from build123d import *

# Parameters (mm, degrees)
BOSS_EXTRU_1_DEPTH = 10
ESQUISSE2_R        = 10
BOSS_EXTRU_2_DEPTH = 110
CONG_1_R           = 2


with BuildPart() as part:
    # Esquisse1 → Boss.-Extru.1 (new body)
    with BuildSketch(Plane(origin=(0, 0, 0), x_dir=(1, 0, 0), z_dir=(0, 1, 0))):
        Polygon((14.736253584, 9.101803684), (-0.514266419, 17.312871803), (-15.250520003, 8.211068118), (-14.736253584, -9.101803684), (0.514266419, -17.312871803), (15.250520003, -8.211068118), align=None)
    extrude(amount=BOSS_EXTRU_1_DEPTH)

    # Esquisse2 → Boss.-Extru.2 (add)
    with BuildSketch(Plane(origin=(0, 10, 0), x_dir=(1, 0, 0), z_dir=(0, 1, 0))):
        Circle(ESQUISSE2_R)
    extrude(amount=BOSS_EXTRU_2_DEPTH)

    # Congé1
    cong_1_edges = [part.edges().sort_by_distance(p)[0] for p in [
        (-10, 120, 0),
    ]]
    fillet(cong_1_edges, radius=CONG_1_R)


solid = part.part
Can you work these out from the model? Positions are in its coordinate system, mm. A direction names the side the tool comes from. Coordinates: 2 decimals unless noted, no trailing zeros. Write each loop counter-clockwise with the first axis right and the second up, starting at its lowest first coordinate (ties: lowest second). Pieces come first, ordered by that corner, then holes. Notation, with made-up numbers: (-15, 31) -> (36, 31) arc R14 cw to (36, 43) -> close; hole circle Ø8 at (25.5, 66.5). An arc over 180 degrees is marked (long way). Write item = value, one per line.
(1) For pin 1 (1.5 mm diameter, centred on y = 80, z = -2, fed in from +X); pin 2 (2 mm diameter, centred on y = 63, z = -8, fed in from +X); pin 3 (12 mm diameter, centred on x = -5, y = 34, fed in from -Z), each with a flat end and sliding along its axis, tell me the tip position at first contact or that it passes through.
Verdict:
pin_1 = 9.92
pin_2 = 7.14
pin_3 = -10
(2) Imagine slicing it at B-B (z = 0). Please give me the cut outline in (x, y), and give its area (3 significant figures).
Verdict:
outline = (-15.01, 0) -> (15.01, 0) -> (15.01, 10) -> (10, 10) -> (10, 118) arc R2 ccw to (8, 120) -> (-8, 120) arc R2 ccw to (-10, 118) -> (-10, 10) -> (-15.01, 10) -> close
area = 2,500 mm^2
(3) Imagine slicing it at C-C (x = -13). Please give me the cut outline in (y, z), and give its area (3 significant figures).
Verdict:
outline = (0, -9.6) -> (10, -9.6) -> (10, 10.04) -> (0, 10.04) -> close
area = 196 mm^2
(4) Imagine slicing it at D-D (x = 13.5). Please give me the cut outline in (y, z).
Verdict:
outline = (0, -9.77) -> (10, -9.77) -> (10, 9.29) -> (0, 9.29) -> close
(5) On a 3-axis mill with a long thin cutter (end or side, diameter ignored), from which of +Z, -Z, +X, -X, +Y, -Y can I reach the whole of each face in a straight line? I mean faces 1 (the face through (7.22, 4.93, -13.15)), 2 (the face through (-7, 10, 7.5)). Say none if no direction works.
Verdict:
face_1 = -Z, +X, +Y, -Y
face_2 = +Y
(6) If I drill on probe 1 along X at (y, z) = (89, 0); probe 2 along Y at (x, z) = (-3.5, -13), over which ranges is the centre line in solid material (lowest first)?
Verdict:
probe_1 = -10 to 10
probe_2 = 0 to 10
(7) Imagine slicing it at A-A (y = 48.5). Please give me the cut outline in (x, z).
Verdict:
outline = circle Ø20 at (0, 0)
